Build history of the part. All positions in model axes, mm. Face numbers are marked on the shaded views. A direction names the side the tool comes from. Give positions to 0.01 mm unless a question says otherwise; leave off trailing zeros. Order: outer loops, then holes, each group sorted by start corner. A loop starts at its lowest first (then second) coordinate and runs counter-clockwise, first axis right, second up. Notation, with made-up numbers: M 58.25,37.25 L 80.25,37.25 A21 ccw 80.25,66.25 Z; hole C 15.5,58 d2. An arc over 180 degrees is marked long. Answer as CSV lines item,"result".
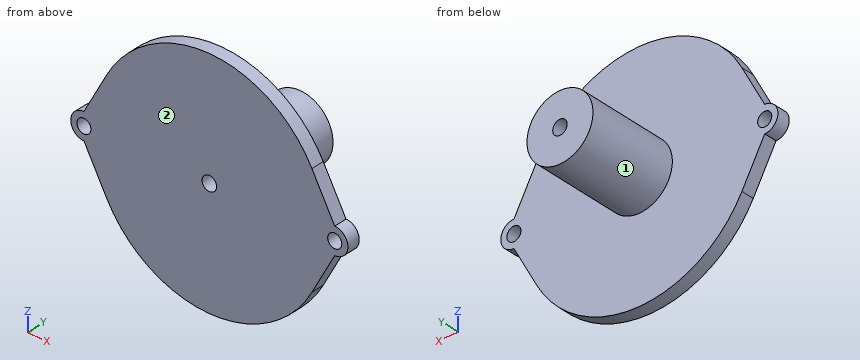
from build123d import *

# Parameters (mm, degrees)
BOSS_EXTRUDE1_DEPTH      = 3
SKETCH2_R                = 7.5
BOSS_EXTRUDE2_DEPTH      = 21
M3_CLEARANCE_HOLE1_D     = 3.2
M3_CLEARANCE_HOLE1_DEPTH = 3
SKETCH5_R                = 1.65
CUT_EXTRUDE1_DEPTH       = 25


with BuildPart() as part:
    # Sketch1 → Boss-Extrude1 (new body)
    with BuildSketch(Plane(origin=(0, 0, 0), x_dir=(1, 0, 0), z_dir=(0, 1, 0))):
        with BuildLine():
            Line((-28.5, 3), (-23.314316453, 12.597327031))
            ThreePointArc((-23.314316453, 12.597327031), (0, 26.5), (23.314316453, 12.597327031))
            Line((23.314316453, 12.597327031), (28.5, 3))
            ThreePointArc((28.5, 3), (31.5, 0), (28.5, -3))
            Line((28.5, -3), (23.314316453, -12.597327031))
            ThreePointArc((23.314316453, -12.597327031), (0, -26.5), (-23.314316453, -12.597327031))
            Line((-23.314316453, -12.597327031), (-28.5, -3))
            ThreePointArc((-28.5, -3), (-31.5, 0), (-28.5, 3))
        make_face()
    extrude(amount=-BOSS_EXTRUDE1_DEPTH)

    # Sketch2 → Boss-Extrude2 (add)
    with BuildSketch(Plane(origin=(0, 0, 0), x_dir=(1, 0, 0), z_dir=(0, 1, 0))):
        Circle(SKETCH2_R)
    extrude(amount=BOSS_EXTRUDE2_DEPTH)

    # M3 Clearance Hole1
    with Locations(Plane(origin=(0, -3, 0), x_dir=(-1, 0, 0), z_dir=(0, -1, 0))):
        with Locations((-28.5, 0), (28.5, 0)):
            Hole(M3_CLEARANCE_HOLE1_D / 2, depth=M3_CLEARANCE_HOLE1_DEPTH)

    # Sketch5 → Cut-Extrude1 (cut, through all)
    with BuildSketch(Plane(origin=(0, 21, 0), x_dir=(1, 0, 0), z_dir=(0, 1, 0))):
        Circle(SKETCH5_R)
    extrude(amount=-CUT_EXTRUDE1_DEPTH, mode=Mode.SUBTRACT)


solid = part.part
Item 1: Probe line 1 along Z through (x, y) = (28.5, -1.8); line 2 along Z through (x, y) = (0, 8.5); line 3 along Y through (x, z) = (-11.5, 16.5). List the from-to ranges inside material, lowest first. Write a range as from..to.
Geometry says:
line 1,"z = -3..-1.6, 1.6..3"
line 2,"z = -7.5..-1.65, 1.65..7.5"
line 3,"y = -3..0"
Item 2: Band-saw the part on B-B (x = 0). Give the cut face in (y, z), and give its area (3 significant figures).
Geometry says:
outline,"M -3,-26.5 L 0,-26.5 L 0,-7.5 L 21,-7.5 L 21,-1.65 L -3,-1.65 Z; M -3,1.65 L 21,1.65 L 21,7.5 L 0,7.5 L 0,26.5 L -3,26.5 Z"
area,"395 mm2"
Item 3: 3-axis set-ups, long thin cutter, end or side, ignore diameter. For the marked faces 1 and 2: which of +Z, -Z, +X, -X, +Y, -Y reach the whole face in a straight line?
Geometry says:
face 1,"+Y"
face 2,"+Z, -Z, +X, -X, -Y"
Item 4: Drop flat-ended pins along their axis: pin 1 (10 mm diameter, centred on y = 1.5, z = 6, fed in from +X); pin 2 (6 mm diameter, centred on x = 23.5, z = -6.5, fed in from +Y); pin 3 (2 mm diameter, centred on y = 14, z = 3.5, fed in from +X); pin 4 (4.5 mm diameter, centred on x = 0, z = 0, fed in from -Y). Give the stop position or say it passes through.
Geometry says:
pin 1,"stops at x = 31.24"
pin 2,"stops at y = 0"
pin 3,"stops at x = 7.07"
pin 4,"stops at y = -3"
Item 5: Band-saw the part on C-C (y = -1.25). Give the cut face in (x, z).
Geometry says:
outline,"M -28.5,-3 L -23.31,-12.6 A26.5 ccw 23.31,-12.6 L 28.5,-3 A3 ccw 28.5,3 L 23.31,12.6 A26.5 ccw -23.31,12.6 L -28.5,3 A3 ccw Z; hole C -28.5,0 d3.2; hole C 0,0 d3.3; hole C 28.5,0 d3.2"
Item 6: Band-saw the part on D-D (y = 15). Give the cut face in (x, z), and give its area (3 significant figures).
Geometry says:
outline,"C 0,0 d15; hole C 0,0 d3.3"
area,"168 mm2"
Item 7: Band-saw the part on A-A (z = 0). Give the cut face in (x, y).
Geometry says:
outline,"M -31.5,-3 L -30.1,-3 L -30.1,0 L -31.5,0 Z; M -26.9,-3 L -1.65,-3 L -1.65,21 L -7.5,21 L -7.5,0 L -26.9,0 Z; M 1.65,-3 L 26.9,-3 L 26.9,0 L 7.5,0 L 7.5,21 L 1.65,21 Z; M 30.1,-3 L 31.5,-3 L 31.5,0 L 30.1,0 Z"
